Input: part model. Units: mm. Frame: model coordinates. Give positions to 0.01 mm unless a question says otherwise; leave off trailing zeros. Loops run counter-clockwise (first coordinate to the right, second up) from the corner with the lowest first, then second, coordinate; pieces in that order, holes last. Notation, with made-up numbers: M 44,6 L 73,6 A22 cw 73,39 Z; hole C 53,68 d6. An arc over 180 degrees is marked long. Answer as a JSON object with one key per item and string values. Group by question number.
1) Section query A-A on x = 55.5. Return loops of the section in (y, z).
2) First-contact query: P1, Ø8, axis at x = 66, y = -8, coming from the +Z side; P2, Ø12, axis at x = 27.5, y = -20, coming from the -Z side. Flat tips, straight axial feed; report the tip coordinate or a pass-through.
3) Section query B-B on y = -7. Return loops of the section in (x, z).
4) Section query C-C on z = 7.5. Count the separate pieces of the cut face and the enclosed holes in it, plus the area to 3 significant figures.
5) Draft query along Y for faces 1 (the flat face through (0, -8, 50)), 2 (the flat face through (-1, -55, 24)), 3 (the flat face through (-1, 9, 26)), 4 (the flat face through (-1, 55, 24)). Return one class per face: +Y half, -Y half, draft (parallel to the pull), parting line (faces both ways), or undercut.
6) Ray query, L1, parallel to X at y = 38, z = 37.5; L2, parallel to Y at x = -47, z = 41.5; L3, parallel to Z at x = -67.5, y = 15. Return the intervals inside material, ascending.
from build123d import *

# Parameters (mm, degrees)
SKETCH001_W     = 170
SKETCH001_H     = 110
PAD_DEPTH       = 50
SKETCH_W        = 82
SKETCH_H        = 16
POCKET_DEPTH    = 48
FILLET_R        = 2
FILLET001_R     = 0.5
SKETCH002_W     = 35
SKETCH002_H     = 90
POCKET001_DEPTH = 50.001


with BuildPart() as part:
    # Sketch001 → Pad (new body)
    with BuildSketch(Plane.XY):
        Rectangle(SKETCH001_W, SKETCH001_H)
    extrude(amount=PAD_DEPTH)

    # Sketch (on Face6 of Pad) → Pocket (cut)
    with BuildSketch(Plane.XY.offset(50)):
        with Locations((-42, 45)):
            Rectangle(SKETCH_W, SKETCH_H)
        with Locations((-42, 27)):
            Rectangle(SKETCH_W, SKETCH_H)
        with Locations((-42, 9)):
            Rectangle(SKETCH_W, SKETCH_H)
        with Locations((42, 45)):
            Rectangle(SKETCH_W, SKETCH_H)
        with Locations((42, 27)):
            Rectangle(SKETCH_W, SKETCH_H)
        with Locations((42, 9)):
            Rectangle(SKETCH_W, SKETCH_H)
        with Locations((-42, -9)):
            Rectangle(SKETCH_W, SKETCH_H)
        with Locations((-42, -27)):
            Rectangle(SKETCH_W, SKETCH_H)
        with Locations((-42, -45)):
            Rectangle(SKETCH_W, SKETCH_H)
        with Locations((42, -9)):
            Rectangle(SKETCH_W, SKETCH_H)
        with Locations((42, -27)):
            Rectangle(SKETCH_W, SKETCH_H)
        with Locations((42, -45)):
            Rectangle(SKETCH_W, SKETCH_H)
    extrude(amount=-POCKET_DEPTH, mode=Mode.SUBTRACT)

    # Fillet
    fillet_edges = [part.edges().sort_by_distance(p)[0] for p in [
        (85, 55, 25),
        (85, -55, 25),
        (-85, -55, 25),
        (-85, 55, 25),
    ]]
    fillet(fillet_edges, radius=FILLET_R)

    # Fillet001
    fillet001_edges = [part.edges().sort_by_distance(p)[0] for p in [
        (0, 55, 50),
        (84.414214, 54.414214, 50),
        (-84.414214, 54.414214, 50),
        (85, 0, 50),
        (-85, 0, 50),
        (84.414214, -54.414214, 50),
        (-84.414214, -54.414214, 50),
        (0, -55, 50),
        (-42, -37, 50),
        (-1, -45, 50),
        (-83, -45, 50),
        (-42, -53, 50),
        (-42, -19, 50),
        (-1, -27, 50),
        (-83, -27, 50),
        (-42, -35, 50),
        (-42, -1, 50),
        (-1, -9, 50),
        (-83, -9, 50),
        (-42, -17, 50),
        (1, -45, 50),
        (42, -53, 50),
        (42, -37, 50),
        (83, -45, 50),
        (1, -27, 50),
        (42, -35, 50),
        (42, -19, 50),
        (83, -27, 50),
        (1, -9, 50),
        (42, -17, 50),
        (42, -1, 50),
        (83, -9, 50),
        (-83, 9, 50),
        (-42, 1, 50),
        (-42, 17, 50),
        (-1, 9, 50),
        (-42, 35, 50),
        (-1, 27, 50),
        (-83, 27, 50),
        (-42, 19, 50),
        (-83, 45, 50),
        (-42, 37, 50),
        (-1, 45, 50),
        (-42, 53, 50),
        (1, 9, 50),
        (42, 1, 50),
        (42, 17, 50),
        (83, 9, 50),
        (1, 27, 50),
        (42, 19, 50),
        (42, 35, 50),
        (83, 27, 50),
        (1, 45, 50),
        (42, 37, 50),
        (42, 53, 50),
        (83, 45, 50),
    ]]
    fillet(fillet001_edges, radius=FILLET001_R)

    # Sketch002 (on Face4 of Fillet001) → Pocket001 (cut, through all)
    with BuildSketch(Plane(origin=(0, 0, 0), x_dir=(1, 0, 0), z_dir=(0, 0, -1))):
        with Locations((-42.5, 0)):
            Rectangle(SKETCH002_W, SKETCH002_H)
        with Locations((42.5, 0)):
            Rectangle(SKETCH002_W, SKETCH002_H)
    extrude(amount=-POCKET001_DEPTH, mode=Mode.SUBTRACT)


solid = part.part
Output:
{
 "1": {"outline": "M -55,0 L -45,0 L -45,2 L -53,2 L -53,49.5 A0.5 ccw -53.5,50 L -54.5,50 A0.5 ccw -55,49.5 Z; M 45,0 L 55,0 L 55,49.5 A0.5 ccw 54.5,50 L 53.5,50 A0.5 ccw 53,49.5 L 53,2 L 45,2 Z"},
 "2": {"P1": "stops at z = 2", "P2": "stops at z = 0"},
 "3": {"outline": "M -85,0 L -60,0 L -60,2 L -83,2 L -83,49.5 A0.5 ccw -83.5,50 L -84.5,50 A0.5 ccw -85,49.5 Z; M -25,0 L 25,0 L 25,2 L 1,2 L 1,49.5 A0.5 ccw 0.5,50 L -0.5,50 A0.5 ccw -1,49.5 L -1,2 L -25,2 Z; M 60,0 L 85,0 L 85,49.5 A0.5 ccw 84.5,50 L 83.5,50 A0.5 ccw 83,49.5 L 83,2 L 60,2 Z"},
 "4": {"separate pieces": "1", "enclosed holes": "2", "area": "2,250 mm^2"},
 "5": {"face 1": "draft", "face 2": "-Y half", "face 3": "undercut", "face 4": "+Y half"},
 "6": {"L1": "x = -85 to -83, -1 to 1, 83 to 85", "L2": "y = -55 to -53, 53 to 55", "L3": "z = 0 to 2"}
}
